The listing builds one solid part. Answer for the finished solid, in the listing's coordinates (mm). Round coordinates to 2 decimals unless told otherwise and drop trailing zeros. Order: outer loops, then holes, each group sorted by start corner. A loop starts at its lowest first (then second) coordinate and runs counter-clockwise, first axis right, second up. Notation, with made-up numbers: (4.5, 57.25) - (16.5, 57.25) arc R33 cw to (16.5, 86.25) - close; hole circle Ø3 at (17.25, 24). An arc over 180 degrees is marked (long way). Write item = value, one per line.
from build123d import *

# Parameters (mm, degrees)
ESQUISSE1_W             = 5.1308
ESQUISSE1_H             = 19.1008
BOSS_EXTRU_1_DEPTH      = 19.05
ENL_V_MAT_EXTRU_1_DEPTH = 20.304
ENL_V_MAT_EXTRU_2_DEPTH = 20.3040001


with BuildPart() as part:
    # Esquisse1 → Boss.-Extru.1 (new body)
    with BuildSketch(Plane(origin=(0, 0, 0), x_dir=(1, 0, 0), z_dir=(0, 1, 0))):
        with Locations((-0.1016, 9.7536)):
            Rectangle(ESQUISSE1_W, ESQUISSE1_H)
    extrude(amount=BOSS_EXTRU_1_DEPTH)

    # Esquisse2 → Enlèv. mat.-Extru.1 (cut, through all)
    with BuildSketch(Plane.XY):
        with BuildLine():
            Line((2.4638, 4.529252061), (2.4638, 0))
            Line((2.4638, 0), (-2.164205313, 0))
            add(Edge.make_bspline(
                [(-2.164205313, 0), (-0.235595225, 2.663077002), (2.4638, 4.529252061)],
                knots=[0, 0, 0, 1, 1, 1], degree=2))
        make_face()
    extrude(amount=-ENL_V_MAT_EXTRU_1_DEPTH, mode=Mode.SUBTRACT)

    # Esquisse3 → Enlèv. mat.-Extru.2 (cut, through all)
    with BuildSketch(Plane.XY):
        with BuildLine():
            Line((-2.667, 18.288), (-2.667, 16.256))
            ThreePointArc((-2.667, 16.256), (-1.651, 17.272), (-2.667, 18.288))
        make_face()
    enl_v_mat_extru_2 = extrude(amount=-ENL_V_MAT_EXTRU_2_DEPTH, mode=Mode.SUBTRACT)

    # Symétrie1: Enlèv. mat.-Extru.2 across plane
    add(enl_v_mat_extru_2.mirror(Plane(origin=(0, 0, 0), x_dir=(0, 0, 1), z_dir=(1, 0, 0))), mode=Mode.SUBTRACT)


solid = part.part
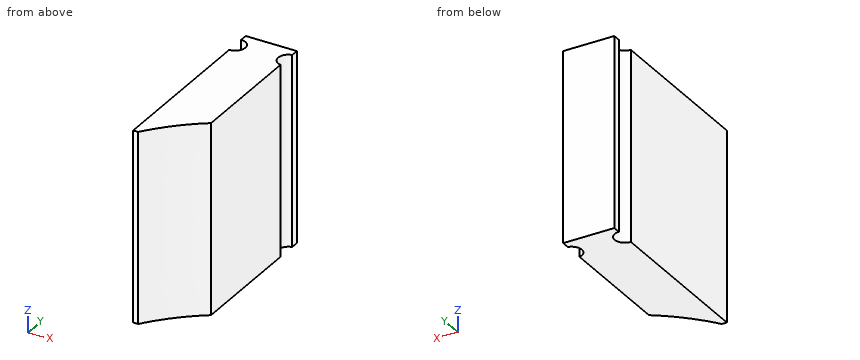
Q1. Find the intervals of material crossed by line 1 (Y direction, x = 1.8, z = -7.5); line 2 (Y direction, x = -2, z = -4); line 3 (Y direction, x = -1.1, z = -3.5), in increasing order. Write a range as from..to.
Model answer:
line_1 = 4.05..16.74, 17.8..19.05
line_2 = 0.22..16.51, 18.04..19.05
line_3 = 1.34..19.05
Q2. Section A-A on y = 16.5 is taken. Determine the outline of the cut face in (x, z).
Model answer:
outline = (-2.01, -19.3) - (2.01, -19.3) - (2.01, -0.2) - (-2.01, -0.2) - close
Q3. A flat-ended cylindrical pin translates along its axis: P1, Ø1.5, axis at x = 0.5, z = -10.5, coming from the -Y side. Find the tip coordinate at first contact, or state that the pin passes through.
Model answer:
P1 = 2.26
